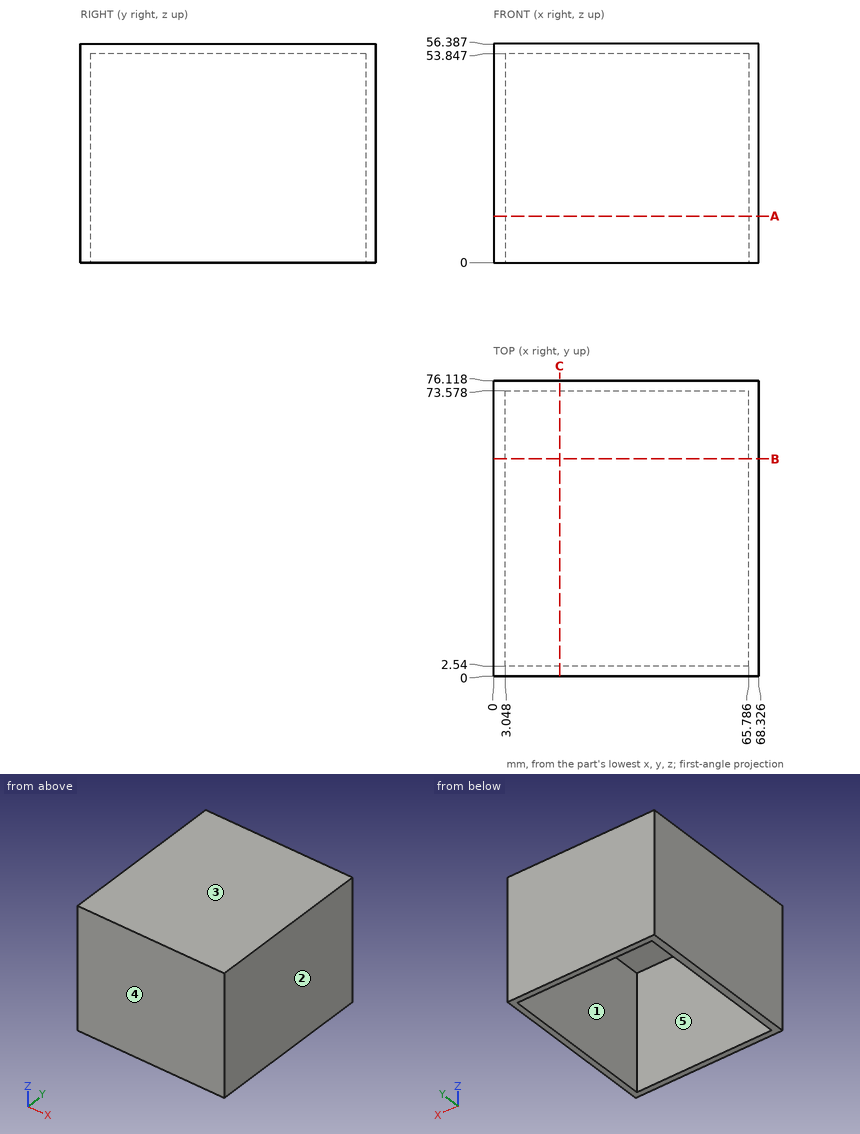
For this review, use the dimensioned drawing (mm, ordinates from the lowest corner) and the shaded views. A direction names the side the tool comes from. Round coordinates to 2 decimals unless told otherwise and drop trailing zeros. Loops run counter-clockwise (first coordinate to the right, second up) from the corner with the lowest first, then second, coordinate; pieces in that order, holes last. Notation, with made-up numbers: M 60,58.25 L 78,58.25 A27 ccw 78,96.25 Z; hole C 75.25,18.25 d9. An arc over 180 degrees is marked long. Answer as a JSON object with one key per item and string values.
(1) Take a section at B-B on y = 56. Give the boundary of the cut face in (x, z).
Resolved:
{"outline": "M 0,0 L 3.05,0 L 3.05,53.85 L 65.79,53.85 L 65.79,0 L 68.33,0 L 68.33,56.39 L 0,56.39 Z"}
(2) Take a section at C-C on x = 17. Give the boundary of the cut face in (y, z), and give its area (3 significant figures).
Resolved:
{"outline": "M 0,0 L 2.54,0 L 2.54,53.85 L 73.58,53.85 L 73.58,0 L 76.12,0 L 76.12,56.39 L 0,56.39 Z", "area": "467 mm²"}
(3) Draft analysis for pull direction Y (two halves, no side actions). For the marked faces 3, 4 and 5, state which applies: released by +Y, released by -Y, zero draft, split by the parting line, or undercut.
Resolved:
{"face 3": "zero draft", "face 4": "released by -Y", "face 5": "undercut"}
(4) Tool access review of the marked faces 1 and 2: name each direction out of +Z, -Z, +X, -X, +Y, -Y from which nothing blocks a thin tool from reaching the whole face with its end or side.
Resolved:
{"face 1": "-Z", "face 2": "+Z, -Z, +X, +Y, -Y"}
(5) To check wall thickness, follow line 1 along Y through (x, z) = (28.5, 53); line 2 along X through (y, z) = (26, 20.5); line 3 along Z through (x, y) = (41.5, 72.5). State the ranges of each line that lie inside material, in increasing order.
Resolved:
{"line 1": "0 to 2.54, 73.58 to 76.12", "line 2": "0 to 3.05, 65.79 to 68.33", "line 3": "53.85 to 56.39"}
(6) Take a section at A-A on z = 12. Give the boundary of the cut face in (x, y), and give its area (3 significant figures).
Resolved:
{"outline": "M 0,0 L 68.33,0 L 68.33,76.12 L 0,76.12 Z; hole M 3.05,2.54 L 65.79,2.54 L 65.79,73.58 L 3.05,73.58 Z", "area": "744 mm²"}
